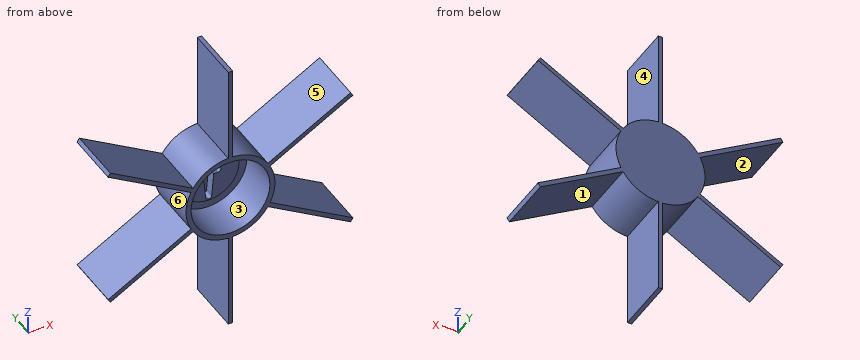
```python
from build123d import *

# Parameters (mm, degrees)
SKETCH_1_R          = 20.5
EXTRUDE_1_DEPTH     = 40
SKETCH_2_R          = 21
EXTRUDE_2_DEPTH     = 35
SKETCH_4_R          = 20.75
CUT_EXTRUDE_2_DEPTH = 28.5
CUT_EXTRUDE_3_DEPTH = 17
EXTRUDE_START       = -40
SKETCH_7_R          = 30.5
SKETCH_7_R_2        = 24.5
EXTRUDE_4_DEPTH     = 40
SKETCH_8_R          = 27
SKETCH_8_R_2        = 20.75
CUT_EXTRUDE_4_DEPTH = 30
SKETCH_9_R          = 20.5
EXTRUDE_5_DEPTH     = 5
SKETCH_11_R         = 155.050037834
CUT_EXTRUDE_5_DEPTH = 1


with BuildPart() as part:
    # 草图1 → 凸台-拉伸1 (new body)
    with BuildSketch(Plane(origin=(0, 0, 0), x_dir=(1, 0, 0), z_dir=(0, 1, 0))):
        with BuildLine():
            Line((82.378289409, -49.293178373), (20.427818585, -13.526057366))
            ThreePointArc((20.427818585, -13.526057366), (12.25, -21.217622393), (1.5, -24.454038521))
            Line((1.5, -24.454038521), (1.5, -95.988280535))
            ThreePointArc((1.5, -95.988280535), (0, -96), (-1.5, -95.988280535))
            Line((-1.5, -95.988280535), (-1.5, -24.454038521))
            ThreePointArc((-1.5, -24.454038521), (-12.25, -21.217622393), (-20.427818585, -13.526057366))
            Line((-20.427818585, -13.526057366), (-82.378289409, -49.293178373))
            ThreePointArc((-82.378289409, -49.293178373), (-83.138438763, -48), (-83.878289409, -46.695102162))
            Line((-83.878289409, -46.695102162), (-21.927818585, -10.927981155))
            ThreePointArc((-21.927818585, -10.927981155), (-24.5, 0), (-21.927818585, 10.927981155))
            Line((-21.927818585, 10.927981155), (-83.878289409, 46.695102162))
            ThreePointArc((-83.878289409, 46.695102162), (-83.138438763, 48), (-82.378289409, 49.293178373))
            Line((-82.378289409, 49.293178373), (-20.427818585, 13.526057366))
            ThreePointArc((-20.427818585, 13.526057366), (-12.25, 21.217622393), (-1.5, 24.454038521))
            Line((-1.5, 24.454038521), (-1.5, 96))
            Line((-1.5, 96), (0.874477385, 96))
            Line((0.874477385, 96), (1.5, 96))
            Line((1.5, 96), (1.5, 24.454038521))
            ThreePointArc((1.5, 24.454038521), (12.25, 21.217622393), (20.427818585, 13.526057366))
            Line((20.427818585, 13.526057366), (82.378289409, 49.293178373))
            ThreePointArc((82.378289409, 49.293178373), (83.138438763, 48), (83.878289409, 46.695102162))
            Line((83.878289409, 46.695102162), (21.927818585, 10.927981155))
            ThreePointArc((21.927818585, 10.927981155), (24.5, 0), (21.927818585, -10.927981155))
            Line((21.927818585, -10.927981155), (83.878289409, -46.695102162))
            ThreePointArc((83.878289409, -46.695102162), (83.138438763, -48), (82.378289409, -49.293178373))
        make_face()
        with Locations(Location((0, 0, 0), (0, 0, 270))):
            Circle(SKETCH_1_R, mode=Mode.SUBTRACT)
    extrude(amount=EXTRUDE_1_DEPTH)

    # 草图2 → 凸台-拉伸2 (add)
    with BuildSketch(Plane.XZ):
        Circle(SKETCH_2_R)
    extrude(amount=-EXTRUDE_2_DEPTH)

    # 草图4 → 切除-拉伸2 (cut)
    with BuildSketch(Plane.XZ):
        with Locations(Location((0, 0, 0), (0, 0, 270))):
            Circle(SKETCH_4_R)
    extrude(amount=-CUT_EXTRUDE_2_DEPTH, mode=Mode.SUBTRACT)

    # 草图6 → 切除-拉伸3 (cut)
    with BuildSketch(Plane.XZ.offset(-28.5)):
        with BuildLine():
            Line((-6.4, 1.95), (-2.9, 1.95))
            Line((-2.9, 1.95), (-2.1, 14.9))
            ThreePointArc((-2.1, 14.9), (0, 17), (2.1, 14.9))
            Line((2.1, 14.9), (2.9, 1.95))
            Line((2.9, 1.95), (6.4, 1.95))
            ThreePointArc((6.4, 1.95), (8.35, 0), (6.4, -1.95))
            Line((6.4, -1.95), (3.5, -1.95))
            Line((3.5, -1.95), (2.1, -17.9))
            ThreePointArc((2.1, -17.9), (0, -20), (-2.1, -17.9))
            Line((-2.1, -17.9), (-3.5, -1.95))
            Line((-3.5, -1.95), (-6.4, -1.95))
            ThreePointArc((-6.4, -1.95), (-8.35, 0), (-6.4, 1.95))
        make_face()
    extrude(amount=-CUT_EXTRUDE_3_DEPTH, mode=Mode.SUBTRACT)

    # 草图7 → 凸台-拉伸4 (add)
    with BuildSketch(Plane(origin=(0, 40, 0), x_dir=(1, 0, 0), z_dir=(0, 1, 0)).offset(EXTRUDE_START)):
        Circle(SKETCH_7_R)
        Circle(SKETCH_7_R_2, mode=Mode.SUBTRACT)
    extrude(amount=EXTRUDE_4_DEPTH)

    # 草图8 → 切除-拉伸4 (cut)
    with BuildSketch(Plane.XZ):
        with Locations(Location((0, 0, 0), (0, 0, 270))):
            Circle(SKETCH_8_R)
        with Locations(Location((0, 0, 0), (0, 0, 270))):
            Circle(SKETCH_8_R_2, mode=Mode.SUBTRACT)
    extrude(amount=-CUT_EXTRUDE_4_DEPTH, mode=Mode.SUBTRACT)

    # 草图9 → 凸台-拉伸5 (add)
    with BuildSketch(Plane(origin=(0, 35, 0), x_dir=(1, 0, 0), z_dir=(0, 1, 0))):
        Circle(SKETCH_9_R)
    extrude(amount=EXTRUDE_5_DEPTH)

    # 草图11 → 切除-拉伸5 (cut)
    with BuildSketch(Plane.XZ):
        Circle(SKETCH_11_R)
    extrude(amount=-CUT_EXTRUDE_5_DEPTH, mode=Mode.SUBTRACT)


solid = part.part
```
Verification items for the finished model (mm, model axes). Face numbers are marked on the shaded views. A direction names the side the tool comes from. Coordinates: 2 decimals unless noted, no trailing zeros. Write each loop counter-clockwise with the first axis right and the second up, starting at its lowest first coordinate (ties: lowest second). Pieces come first, ordered by that corner, then holes. Notation, with made-up numbers: (-25, -38.5) - (0, -38.5) arc R22 cw to (0, -7.5) - close; hole circle Ø10 at (38.25, 43). An arc over 180 degrees is marked (long way). One line per question, with ' | ' between items. Start each with the question number.
1. Draft check along Z on the marked faces 4, 5 and 6. Enter one of: released by +Z, released by -Z, zero draft, split by the parting line, or undercut.
2. Section check C-C (z = -75). Enter the section's corners in (x, y).
3. Gauge pin test, flat ends, axial feed: P1, Ø2.5, axis at x = -4.5, y = 32.5, coming from the +Z side; P2, Ø11.5, axis at y = 12, z = 58.5, coming from the -X side; P3, Ø5, axis at x = -31, y = 14.5, coming from the +Z side. Record the tip position at first contact, or that the pin passes through.
4. Section check A-A (y = 14). Enter the section's corners in (x, z).
5. Access from +Z, -Z, +X, -X, +Y, -Y to the whole of each face (thin tool, end or side, straight path). Record for the marked faces 1, 2 and 3.
6. Material ranges on line 1 along X through (y, z) = (9.25, 0); line 2 along X through (y, z) = (5.5, -17.5); line 3 along Z through (x, y) = (63, 12), recorded low to high.
7. Section check B-B (x = 48.5). Enter the section's corners in (y, z).
Computed values:
1) face 4: zero draft | face 5: released by +Z | face 6: undercut
2) outline: (-1.5, 1) - (1.5, 1) - (1.5, 40) - (-1.5, 40) - close
3) P1: z = 30.33 | P2: x = -1.5 | P3: z = 21.07
4) outline: (-83.88, -46.7) arc R96 ccw to (-82.38, -49.29) - (-25.63, -16.53) arc R30.5 ccw to (-1.5, -30.46) - (-1.5, -96) - (1.5, -96) - (1.5, -30.46) arc R30.5 ccw to (25.63, -16.53) - (82.38, -49.29) arc R96 ccw to (83.88, -46.7) - (27.13, -13.93) arc R30.5 ccw to (27.13, 13.93) - (83.88, 46.7) arc R96 ccw to (82.38, 49.29) - (25.63, 16.53) arc R30.5 ccw to (1.5, 30.46) - (1.5, 95.99) arc R96 ccw to (-1.5, 95.99) - (-1.5, 30.46) arc R30.5 ccw to (-25.63, 16.53) - (-82.38, 49.29) arc R96 ccw to (-83.88, 46.7) - (-27.13, 13.93) arc R30.5 ccw to (-27.13, -13.93) - close; hole circle Ø54 at (0, 0)
5) face 1: -Z, +Y, -Y | face 2: -X, +Y, -Y | face 3: -Y
6) line 1: -30.5 to -27, 27 to 30.5 | line 2: -33.31 to -27.31, -24.98 to -20.56, 20.56 to 24.98, 27.31 to 33.31 | line 3: -38.11 to -34.64, 34.64 to 38.11
7) outline: (1, -29.73) - (40, -29.73) - (40, -26.27) - (1, -26.27) - close; (1, 26.27) - (40, 26.27) - (40, 29.73) - (1, 29.73) - close
